CAD build for the part. Positions are in the model's coordinates, mm. A direction names the side the tool comes from. Round coordinates to 2 decimals unless told otherwise and drop trailing zeros. Answer as CSV lines item,"result". Start each with the question number.
from build123d import *

# Parameters (mm, degrees)
ESQUISSE1_R             = 6
BOSS_EXTRU_1_DEPTH      = 10
FILETAGE1_PITCH         = 1.4
FILETAGE1_FROM          = 1
ESQUISSE23_R            = 2.5
ENL_V_MAT_EXTRU_1_DEPTH = 5.5
ESQUISSE24_R            = 1
ENL_V_MAT_EXTRU_2_DEPTH = 3


with BuildPart() as part:
    # Esquisse1 → Boss.-Extru.1 (new body)
    with BuildSketch(Plane(origin=(0, 0, 0), x_dir=(1, 0, 0), z_dir=(0, 1, 0))):
        with Locations(Location((0, 0, 0), (0, 0, 270))):
            Circle(ESQUISSE1_R)
    extrude(amount=BOSS_EXTRU_1_DEPTH)

    # Filetage1: arcs per turn and ends read off the stored shape
    # Filetage1: the profile of Profil de filetage2 profile screwed along a right-hand helix through 7 turns, 8 arcs to a turn; built about Z, then put on its axis
    filetage1_z = Axis((0, 0, 0), (0, 0, 1))
    filetage1_corners = [(5.9997, 0, -0.000173205), (6.811898812, 0, 0.468749998), (6.811898812, 0, 0.656249998), (5.9997, 0, 1.125173201)]
    with BuildLine(mode=Mode.PRIVATE) as filetage1_profile:
        Line(filetage1_corners[0], filetage1_corners[1])
        Line(filetage1_corners[1], filetage1_corners[2])
        Line(filetage1_corners[2], filetage1_corners[3])
        Line(filetage1_corners[3], filetage1_corners[0])
    filetage1_cap = Face(filetage1_profile.wire())
    filetage1_turn_angles = [0, 22.5, 45, 67.5, 90, 112.5, 135, 157.5, 180, 202.5, 225, 247.5, 270, 292.5, 315, 337.5, 360]
    filetage1_turn_weights = [1, 0.9238795325112867, 1, 0.9238795325112867, 1, 0.9238795325112867, 1, 0.9238795325112867, 1, 0.9238795325112867, 1, 0.9238795325112867, 1, 0.9238795325112867, 1, 0.9238795325112867, 1]
    filetage1_turn_rails = [Edge.make_bspline([Vector(p[0], p[1], 0).rotate(filetage1_z, filetage1_turn_angles[k]) / filetage1_turn_weights[k] + Vector(0, 0, p[2] + FILETAGE1_PITCH * filetage1_turn_angles[k] / 360) for k in range(17)], [0, 0, 0, 1, 1, 2, 2, 3, 3, 4, 4, 5, 5, 6, 6, 7, 7, 8, 8, 8], 2, filetage1_turn_weights) for p in filetage1_corners]
    filetage1_turn_sides = [Face.make_surface_from_curves(filetage1_turn_rails[p[0]], filetage1_turn_rails[p[1]]) for p in [(0, 1), (1, 2), (2, 3), (3, 0)]]
    filetage1 = Plane(origin=(0, -1, 0), x_dir=(1, 0, 0), z_dir=(0, 1, 0)) * split(Solid(Shell([*[p.moved(Location((0, 0, FILETAGE1_PITCH * i))) for i in range(7) for p in filetage1_turn_sides], filetage1_cap, filetage1_cap.rotate(filetage1_z, 2520).moved(Location((0, 0, FILETAGE1_PITCH * 2520 / 360)))])), bisect_by=Plane.XY.offset(FILETAGE1_FROM), keep=Keep.TOP, mode=Mode.PRIVATE)
    add(filetage1)

    # Esquisse23 → Enlèv. mat.-Extru.1 (cut)
    with BuildSketch(Plane(origin=(0, 10, 0), x_dir=(1, 0, 0), z_dir=(0, 1, 0))):
        with Locations(Location((0, 0, 0), (0, 0, 270))):
            Circle(ESQUISSE23_R)
    extrude(amount=-ENL_V_MAT_EXTRU_1_DEPTH, mode=Mode.SUBTRACT)

    # Esquisse24 → Enlèv. mat.-Extru.2 (cut)
    with BuildSketch(Plane(origin=(0, 10, 0), x_dir=(1, 0, 0), z_dir=(0, 1, 0))):
        with Locations(Location((4.25, 0, 0), (0, 0, 270))):
            Circle(ESQUISSE24_R)
        with Locations(Location((-4.25, 0, 0), (0, 0, 270))):
            Circle(ESQUISSE24_R)
    extrude(amount=-ENL_V_MAT_EXTRU_2_DEPTH, mode=Mode.SUBTRACT)


solid = part.part
Item 1: Probe line 1 (Y direction, x = 4.5, z = -0.25); line 2 (X direction, y = 6.5, z = -0.25); line 3 (X direction, y = 2, z = -3.75). List the from-to ranges inside material, lowest first.
Item 2: Mould opens along Z. For faces 3 (the cylindrical face through (5.24, 8.52, -0.13)), 4 (the flat face through (0, 0, 0)), 5 (the flat face through (6.3, 9.4, 0)) say: released by +Z, released by -Z, zero draft, split by the parting line, or undercut.
Item 3: Pin check, flat tips, straight feed: pin 1 (2 mm diameter, centred on y = 7.5, z = 2.5, fed in from +X); pin 2 (4.5 mm diameter, centred on x = 0, z = 0, fed in from +Y); pin 3 (4 mm diameter, centred on y = 8, z = -3.5, fed in from -X). Stop position of each tip, or through.
Item 4: Tool access for faces 1 (the flat face through (0, 10, 3)), 2 (the flat face through (4, 7, 0)): list every direction of +Z, -Z, +X, -X, +Y, -Y with a clear straight run to the whole face (end or side of a thin tool).
Values:
1,line 1,"0 to 7"
1,line 2,"-5.99 to -2.49, 2.49 to 6.81"
1,line 3,"-4.85 to 4.8"
2,face 3,"undercut"
2,face 4,"zero draft"
2,face 5,"released by -Z"
3,pin 1,"x = 6.63"
3,pin 2,"y = 4.5"
3,pin 3,"x = -6.63"
4,face 1,"+Z, -Z, +X, -X, +Y"
4,face 2,"+Y"
